For this review, take the finished solid that the model builds, in its own axes (mm). Face numbers are marked on the shaded views. A direction names the side the tool comes from. Round coordinates to 2 decimals unless told otherwise and drop trailing zeros. Order: outer loops, then holes, each group sorted by start corner. A loop starts at its lowest first (then second) coordinate and runs counter-clockwise, first axis right, second up. Notation, with made-up numbers: (63, -2) - (81, -2) arc R23 ccw to (81, 15) - close; hole circle Ø7 at (-8.5, 52.5). An arc over 180 degrees is marked (long way). Write each question's results on one line, items separated by ' | '. Start each with the question number.
(1) Draft analysis for pull direction Y (two halves, no side actions). For the marked faces 1, 2, 3 and 4, state which applies: pulls with the +Y half, pulls with the -Y half, needs draft (parallel to the pull), parting line crosses it, or undercut.
(2) Take a section at B-B, the plane y = 21. Give the boundary of the cut face in (x, z), plus the area to 3 significant figures.
(3) For the marked faces 5, 6, 7 and 8, list the 3-axis set-ups (+Z, -Z, +X, -X, +Y, -Y) from which the entire face can be reached by the end or side of a thin tool; tool diameter is ignored.
(4) For L1, parallel to Y at x = 10.8, z = -5.6; L2, parallel to Z at x = 7.5, y = 0; L3, parallel to Z at x = 7.5, y = 17, list the stretches that pass through material, from the lowest coordinate up. Write a range as from..to.
(5) Insertion check: pin 1 Ø2 at (x, z) = (-11.5, -2.5) entering from +Y; pin 2 Ø2.5 at (x, z) = (-1.5, -1) entering from -Y; pin 3 Ø1.4 at (y, z) = (24, -1) entering from +X; pin 4 Ø3 at (x, y) = (-1.5, 8.5) entering from +Z. Each pin has a flat end and moves straight along its axis. Give the tip position at first contact, or say it passes through.
(6) Take a section at A-A, the plane x = -0.5. Give the boundary of the cut face in (y, z) (3 decimals), plus the area to 3 significant figures.
(7) Take a section at C-C, the plane y = 4.25. Give the boundary of the cut face in (x, z) (3 decimals).
Autodesk Inventor part; units mm, degrees
ref_plane "YZ Plane" through (0, 0, 0) normal (1, 0, 0) x (0, 1, 0)
ref_plane "XZ Plane" through (0, 0, 0) normal (0, 1, 0) x (-1, 0, 0)
ref_plane "XY Plane" through (0, 0, 0) normal (0, 0, 1) x (1, 0, 0)
sketch "Sketch1" plane through (0, 0, 0) normal (0, 0, 1) x (1, 0, 0)
  line L0 (-5, -2.5) -> (5, -2.5) construction
  line L1 (5, -2.5) -> (12.675, 0) construction
  line L2 (-5, -2.5) -> (-12.675, 0)
  line L3 (12.675, 0) -> (-12.675, 0) construction
  line L4 (12.675, 0) -> (12.675, 8.7) construction
  line L5 (-12.675, 0) -> (-12.675, 8.7)
  line L6 (-12.675, 8.7) -> (-4.75, 23.2)
  line L7 (-4.75, 23.2) -> (-4.75, 25.7)
  line L8 (-4.75, 25.7) -> (4.75, 25.7) construction
  line L9 (4.75, 25.7) -> (4.75, 23.2) construction
  line L10 (4.75, 23.2) -> (12.675, 8.7) construction
  line L11 (0, -8.56) -> (0, 31.76)
  line L12 (0, 25.7) -> (0, -2.5)
  circle A0 centre (-10.8, 4.25) radius 1.25
  line L13 (-10.8, 4.25) -> (0, 4.25) construction
  line L14 (-4.75, 25.7) -> (0, 25.7)
  line L15 (-5, -2.5) -> (0, -2.5)
  line L16 (-5.05, 23.2766) -> (-12.975, 8.7766)
  line L17 (-12.975, 8.7766) -> (-12.975, -0.2178)
  line L18 (-12.975, -0.2178) -> (-5.0476, -2.8)
  line L19 (-5.0476, -2.8) -> (0.3, -2.8) construction
  line L20 (0.3, -2.8) -> (0.3, 26) construction
  line L21 (0.3, 26) -> (-5.05, 26) construction
  line L22 (-5.05, 26) -> (-5.05, 23.2766)
  line L23 (0, -2.5) -> (0, -2.8)
  line L24 (0, 25.7) -> (0, 26)
  line L25 (0, -2.8) -> (-5.0476, -2.8)
  line L26 (0, 26) -> (-5.05, 26)
  point P0 (0, 0)
  point P1 (0, 0)
  dimension "d0" = 10
  dimension "d1" = 25.35
  dimension "d2" = 2.5
  dimension "d3" = 8.7
  dimension "d4" = 28.2
  dimension "d6" = 2.5
  dimension "d7" = 9.5
  dimension "d42" = 2.5
  dimension "d43" = 10.8
  dimension "d44" = 6.75
  dimension "d53" = 0.3
sketch "Sketch8" plane through (0, 0, 0) normal (0, 0, 1) x (1, 0, 0)
  line L0 (-20, 30) -> (20, 30)
  line L1 (20, 30) -> (20, -10)
  line L2 (20, -10) -> (-20, -10)
  line L3 (-20, -10) -> (-20, 30)
  point P0 (0, 0)
  point P1 (0, -10)
  dimension "d45" = 40
  dimension "d46" = 10
extrude "MainBlock" add sketch "Sketch8" against normal blind 7
extrude "CartridgeCutout" cut sketch "Sketch1" against normal blind 3
sketch "Sketch10" plane through (-10.8, 4.25, 0) normal (0, 0, 1) x (1, 0, 0)
  circle A0 centre (0, 0) radius 1.25
  circle A1 centre (0, 0) radius 1.45
  point P0 (10.8, -4.25)
  dimension "d56" = 0.2
extrude "PinHole" cut sketch "Sketch10" against normal through all contours A0 | A1
mirror "Mirror3" about plane through (0, 26, 0) normal (-1, 0, 0) of "CartridgeCutout", "PinHole"
sketch "Sketch12" plane through (0, 0, -3) normal (0, 0, 1) x (1, 0, 0)
  circle A0 centre (10.8, 4.25) radius 1.45
  circle A1 centre (-10.8, 4.25) radius 1.45
  line L0 (5.05, 26) -> (-5.05, 26)
  line L1 (-5.05, 23.2766) -> (-5.05, 26)
  line L2 (-12.975, 8.7766) -> (-5.05, 23.2766)
  line L3 (-12.975, -0.2178) -> (-12.975, 8.7766)
  line L4 (-5.0476, -2.8) -> (-12.975, -0.2178)
  line L5 (5.0476, -2.8) -> (-5.0476, -2.8)
  line L6 (5.0476, -2.8) -> (12.975, -0.2178)
  line L7 (12.975, -0.2178) -> (12.975, 8.7766)
  line L8 (12.975, 8.7766) -> (5.05, 23.2766)
  line L9 (5.05, 23.2766) -> (5.05, 26)
  line L10 (-4.15, 23.6) -> (4.15, 23.6)
  line L11 (4.15, 23.6) -> (4.15, -1.4)
  line L12 (4.15, -1.4) -> (-4.15, -1.4)
  line L13 (-4.15, -1.4) -> (-4.15, 23.6)
  point P0 (0, 0)
  point P1 (0, -1.4)
  dimension "d59" = 8.3
  dimension "d60" = 25
  dimension "d61" = 1.4
extrude "CentreHole" cut sketch "Sketch12" against normal through all contours L10 L11 L12 L13
sketch "Sketch13" plane through (0, 0, 0) normal (0, 0, 1) x (1, 0, 0)
  line L0 (-5.05, 26) -> (5.05, 26)
  line L1 (5.05, 26) -> (5.05, 23.2766)
  line L2 (5.05, 23.2766) -> (12.975, 8.7766)
  line L3 (12.975, 8.7766) -> (12.975, -0.2178)
  line L4 (12.975, -0.2178) -> (5.0476, -2.8)
  line L5 (5.0476, -2.8) -> (-5.0476, -2.8)
  line L6 (-5.0476, -2.8) -> (-12.975, -0.2178)
  line L7 (-12.975, -0.2178) -> (-12.975, 8.7766)
  line L8 (-12.975, 8.7766) -> (-5.05, 23.2766)
  line L9 (-5.05, 23.2766) -> (-5.05, 26)
  line L10 (-20, 30) -> (20, 30)
  line L11 (-20, -10) -> (-20, 30)
  line L12 (20, -10) -> (-20, -10)
  line L13 (20, 30) -> (20, -10)
  line L14 (-17, 9.8048) -> (-17, -3.1399)
  line L15 (-17, -3.1399) -> (-5.6866, -6.825)
  line L16 (-5.6866, -6.825) -> (5.6866, -6.825)
  line L17 (5.6866, -6.825) -> (17, -3.1399)
  line L18 (17, -3.1399) -> (17, 9.8048)
  line L19 (17, 9.8048) -> (9.075, 24.3048)
  line L20 (9.075, 24.3048) -> (9.075, 30.025)
  line L21 (9.075, 30.025) -> (-9.075, 30.025)
  line L22 (-9.075, 30.025) -> (-9.075, 24.3048)
  line L23 (-9.075, 24.3048) -> (-17, 9.8048)
  point P0 (0, 0)
  dimension "d65" = 4.025
extrude "OutlineCut" cut sketch "Sketch13" against normal through all contours L10 L22 L23 L14 L15 L16 L17 L18 L19 L20 L13 L12 L11
sketch "Sketch14" plane through (0, 0, -3) normal (0, 0, 1) x (1, 0, 0)
  line L0 (-4.15, -1.4) -> (-4.15, 23.6)
  line L1 (-4.15, 23.6) -> (4.15, 23.6)
  line L2 (4.15, 23.6) -> (4.15, -1.4)
  line L3 (4.15, -1.4) -> (-4.15, -1.4) construction
  circle A0 centre (10.8, 4.25) radius 1.45 construction
  circle A1 centre (-10.8, 4.25) radius 1.45 construction
  line L4 (5.05, 26) -> (-5.05, 26)
  line L5 (-5.05, 23.2766) -> (-5.05, 26)
  line L6 (-12.975, 8.7766) -> (-5.05, 23.2766)
  line L7 (-12.975, -0.2178) -> (-12.975, 8.7766) construction
  line L8 (-5.0476, -2.8) -> (-12.975, -0.2178) construction
  line L9 (5.0476, -2.8) -> (-5.0476, -2.8) construction
  line L10 (5.0476, -2.8) -> (12.975, -0.2178) construction
  line L11 (12.975, -0.2178) -> (12.975, 8.7766) construction
  line L12 (12.975, 8.7766) -> (5.05, 23.2766)
  line L13 (5.05, 23.2766) -> (5.05, 26)
  line L14 (-9.7922, 14.6) -> (-4.15, 14.6)
  line L15 (-12.975, 8.7766) -> (-5.05, 23.2766)
  line L16 (-4.15, 23.6) -> (-5.05, 23.2766)
  line L17 (0, -18) -> (0, 38)
  line L18 (-4.15, 23.6) -> (-4.15, 14.6)
  line L19 (-4.15, -1.4) -> (-4.15, 23.6)
  line L20 (-5.05, 23.2766) -> (-9.7922, 14.6)
  line L21 (-12.975, 8.7766) -> (-5.05, 23.2766)
  line L22 (9.7922, 14.6) -> (4.15, 14.6)
  line L23 (4.15, 23.6) -> (5.05, 23.2766)
  line L24 (4.15, 23.6) -> (4.15, 14.6)
  line L25 (5.05, 23.2766) -> (9.7922, 14.6)
  point P0 (0, 0)
  dimension "d70" = 9
extrude "AlignmentGooveCut" cut sketch "Sketch14" against normal blind 1 contours L14 L6 L16 L0 | L23 L12 L22 L2
sketch "Sketch16" plane through (0, 0, 0) normal (0, 0, 1) x (1, 0, 0)
  line L0 (-8.5, 12.6) -> (8.5, 12.6)
  line L1 (8.5, 12.6) -> (8.5, -7.4)
  line L2 (8.5, -7.4) -> (-8.5, -7.4)
  line L3 (-8.5, -7.4) -> (-8.5, 12.6)
  line L4 (4.15, -1.4) -> (-4.15, -1.4)
  point P0 (0, 0)
  point P1 (0, -7.4)
  dimension "d73" = 17
  dimension "d74" = 20
  dimension "d75" = 14
extrude "CircuitBoardCut" cut sketch "Sketch16" against normal blind 6
fillet "Fillet3" radius 1 10 edges at (-17, -3.1399, -3.5) (17, -3.1399, -3.5) (17, 9.8048, -3.5) (9.075, 24.3048, -3.5) (9.075, 30, -3.5) (-9.075, 24.3048, -3.5) (-17, 9.8048, -3.5) (-9.075, 30, -3.5) (-8.5, -5.9086, -3) (8.5, -5.9086, -3)
fillet "Fillet3" radius 1 2 edges at (-8.5, 12.6, -4.5) (8.5, 12.6, -4.5)
properties part number "InkjetHolderV4"
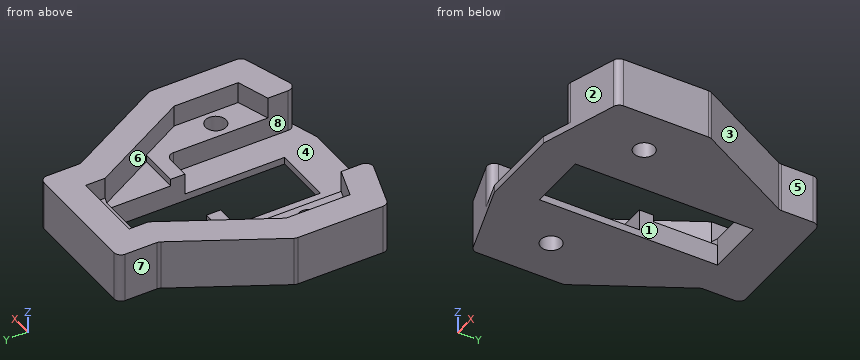
Results below:
1) face 1: undercut | face 2: pulls with the -Y half | face 3: pulls with the +Y half | face 4: needs draft
2) outline: (-10.88, -7) - (-4.15, -7) - (-4.15, -4) - (-6.29, -4) - (-6.29, 0) - (-10.88, 0) - close; (4.15, -7) - (10.88, -7) - (10.88, 0) - (6.29, 0) - (6.29, -4) - (4.15, -4) - close | area: 77.1 mm^2
3) face 5: +Z, -Z, +X, +Y | face 6: +Z | face 7: +Z, -Z, -X, +Y | face 8: +Z, -Y
4) L1: y = -5.16..2.8, 5.7..21.15 | L2: z = -7..-6 | L3: z = -7..-4
5) pin 1: stops at y = 21.7 | pin 2: stops at y = 26 | pin 3: stops at x = 9.62 | pin 4: passes through
6) outline: (-6.825, -7) - (-1.4, -7) - (-1.4, -6) - (-6.825, -6) - close; (23.6, -7) - (30, -7) - (30, 0) - (26, 0) - (26, -3) - (23.6, -3) - close | area: 43.0 mm^2
7) outline: (-17, -7) - (-12.25, -7) - (-12.25, -3) - (-12.975, -3) - (-12.975, 0) - (-17, 0) - close; (-9.35, -7) - (-4.15, -7) - (-4.15, -6) - (-8.5, -6) - (-8.5, -3) - (-9.35, -3) - close; (4.15, -7) - (9.35, -7) - (9.35, -3) - (8.5, -3) - (8.5, -6) - (4.15, -6) - close; (12.25, -7) - (17, -7) - (17, 0) - (12.975, 0) - (12.975, -3) - (12.25, -3) - close
